```python
from build123d import *

# Parameters (mm, degrees)
SKETCH1_W           = 50
SKETCH1_H           = 37
BOSS_EXTRUDE1_DEPTH = 4
CHAMFER1_SIZE       = 10
SKETCH2_W           = 6
SKETCH2_H           = 37
BOSS_EXTRUDE2_DEPTH = 6
SKETCH3_W           = 37
SKETCH3_H           = 4
BOSS_EXTRUDE3_DEPTH = 40
FILLET1_R           = 10
SKETCH4_R           = 2
CUT_EXTRUDE1_DEPTH  = 40
SKETCH5_R           = 3.25
CUT_EXTRUDE2_DEPTH  = 40
SKETCH6_R           = 7.5
CUT_EXTRUDE3_DEPTH  = 5
SKETCH7_R           = 1.5
CUT_EXTRUDE4_DEPTH  = 9
FILLET2_R           = 2


with BuildPart() as part:
    # Sketch1 → Boss-Extrude1 (new body)
    with BuildSketch(Plane(origin=(0, 0, 0), x_dir=(1, 0, 0), z_dir=(0, 1, 0))):
        Rectangle(SKETCH1_W, SKETCH1_H)
    extrude(amount=BOSS_EXTRUDE1_DEPTH)

    # Chamfer1
    chamfer1_edges = [part.edges().sort_by_distance(p)[0] for p in [
        (-25, 2, 18.5),
        (-25, 2, -18.5),
    ]]
    chamfer(chamfer1_edges, length=CHAMFER1_SIZE)

    # Sketch2 → Boss-Extrude2 (add)
    with BuildSketch(Plane(origin=(0, 4, 0), x_dir=(1, 0, 0), z_dir=(0, 1, 0))):
        with Locations((22, 0)):
            Rectangle(SKETCH2_W, SKETCH2_H)
    extrude(amount=BOSS_EXTRUDE2_DEPTH)

    # Sketch3 → Boss-Extrude3 (add)
    with BuildSketch(Plane.ZY.offset(-19)):
        with Locations((0, 8)):
            Rectangle(SKETCH3_W, SKETCH3_H)
    extrude(amount=BOSS_EXTRUDE3_DEPTH)

    # Fillet1
    fillet1_edges = [part.edges().sort_by_distance(p)[0] for p in [
        (-21, 8, -18.5),
        (-21, 8, 18.5),
    ]]
    fillet(fillet1_edges, radius=FILLET1_R)

    # Sketch4 → Cut-Extrude1 (cut)
    with BuildSketch(Plane(origin=(0, 10, 0), x_dir=(1, 0, 0), z_dir=(0, 1, 0))):
        with Locations(Location((-9, -8.5, 0), (0, 0, 270))):
            Circle(SKETCH4_R)
        with Locations(Location((-9, 8.5, 0), (0, 0, 270))):
            Circle(SKETCH4_R)
    extrude(amount=-CUT_EXTRUDE1_DEPTH, mode=Mode.SUBTRACT)

    # Sketch5 → Cut-Extrude2 (cut)
    with BuildSketch(Plane(origin=(0, 10, 0), x_dir=(1, 0, 0), z_dir=(0, 1, 0))):
        with Locations(Location((8.102581703, 0, 0), (0, 0, 270))):
            Circle(SKETCH5_R)
    extrude(amount=-CUT_EXTRUDE2_DEPTH, mode=Mode.SUBTRACT)

    # Sketch6 → Cut-Extrude3 (cut)
    with BuildSketch(Plane.XZ):
        with Locations(Location((8.102581703, 0, 0), (0, 0, 270))):
            Circle(SKETCH6_R)
    extrude(amount=-CUT_EXTRUDE3_DEPTH, mode=Mode.SUBTRACT)

    # Sketch7 → Cut-Extrude4 (cut)
    with BuildSketch(Plane(origin=(0, 10, 0), x_dir=(1, 0, 0), z_dir=(0, 1, 0))):
        with Locations(Location((22.2, 13.5, 0), (0, 0, 270))):
            Circle(SKETCH7_R)
        with Locations(Location((22.2, 4.5, 0), (0, 0, 270))):
            Circle(SKETCH7_R)
        with Locations(Location((22.2, -4.5, 0), (0, 0, 270))):
            Circle(SKETCH7_R)
        with Locations(Location((22.2, -13.5, 0), (0, 0, 270))):
            Circle(SKETCH7_R)
    extrude(amount=-CUT_EXTRUDE4_DEPTH, mode=Mode.SUBTRACT)

    # Fillet2
    fillet2_edges = [part.edges().sort_by_distance(p)[0] for p in [
        (25, 5, 18.5),
        (25, 5, -18.5),
    ]]
    fillet(fillet2_edges, radius=FILLET2_R)


solid = part.part
```
Check sheet for the modelled part. Datum: model origin and axes. Units: mm. A direction names the side the tool comes from. Coordinates: 2 decimals unless noted, no trailing zeros. Order: outer loops, then holes, each group sorted by start corner. A loop starts at its lowest first (then second) coordinate and runs counter-clockwise, first axis right, second up. Notation, with made-up numbers: (-40, 22.5) -> (4, 22.5) arc R21 ccw to (4, 31.5) -> close; hole circle Ø1 at (10.25, 69). An arc over 180 degrees is marked (long way). Write item = value, one per line. Start each with the question number.
1) Cross-section at C-C (y = 2.25). Enter the section's corners in (x, z).
2) Mould release check, pull along Z, two halves, no side actions. Record for faces 1 (the flat face through (0, 0, 0)), 2 (the cylindrical face through (23.465, 5.563, 5.306)), 3 (the cylindrical face through (24.4, 4.93, -17.93)), 4 (the flat face through (4.3, 3.8, 18.5)): +Z half, -Z half, draft (parallel to the pull), parting line (faces both ways), or undercut.
3) Go/stop test with flat-tipped pins: P1, Ø6, axis at y = 8.5, z = 8.5, coming from the -X side; P2, Ø1, axis at x = 5.5, z = 5, coming from the -Y side; P3, Ø1, axis at y = 5, z = 3, coming from the -X side; P4, Ø6.5, axis at x = -9, z = 8.5, coming from the -Y side. Record where each tip stops, or that it passes through.
4) Cross-section at B-B (z = 4.5). Enter the section's corners in (x, y).
5) Cross-section at D-D (z = -1.5). Enter the section's corners in (x, y), then the cut area to 3 significant figures.
6) Cross-section at A-A (x = -9). Enter the section's corners in (y, z), then the cut area to 3 significant figures.
7) Access from +Z, -Z, +X, -X, +Y, -Y to the whole of each face (thin tool, end or side, straight path). Record for faces 5 (the cylindrical face through (-17.99, 8.03, -15.65)), 6 (the flat face through (22, 1, 13)), 7 (the cylindrical face through (15.54, 1.97, 0.98)), 8 (the flat face through (-1, 6, 0)).
8) Material ranges on L1, parallel to X at y = 1.7, z = 0; L2, parallel to Y at x = -1, z = 3; L3, parallel to X at y = 2.1, z = 8.5, recorded low to high.
Ans:
q1.outline = (-25, -8.5) -> (-15, -18.5) -> (23, -18.5) arc R2 ccw to (25, -16.5) -> (25, 16.5) arc R2 ccw to (23, 18.5) -> (-15, 18.5) -> (-25, 8.5) -> close; hole circle Ø4 at (-9, -8.5); hole circle Ø4 at (-9, 8.5); hole circle Ø15 at (8.1, 0); hole circle Ø3 at (22.2, -13.5); hole circle Ø3 at (22.2, -4.5); hole circle Ø3 at (22.2, 4.5); hole circle Ø3 at (22.2, 13.5)
q2.face_1 = draft
q2.face_2 = undercut
q2.face_3 = -Z half
q2.face_4 = +Z half
q3.P1 = -21
q3.P2 = 6
q3.P3 = 19
q3.P4 = 0
q4.outline = (-25, 0) -> (2.1, 0) -> (2.1, 4) -> (-25, 4) -> close; (-21, 6) -> (19, 6) -> (19, 4) -> (14.1, 4) -> (14.1, 0) -> (25, 0) -> (25, 10) -> (23.7, 10) -> (23.7, 1) -> (20.7, 1) -> (20.7, 10) -> (-21, 10) -> close
q5.outline = (-25, 0) -> (0.75, 0) -> (0.75, 4) -> (-25, 4) -> close; (-21, 6) -> (5.22, 6) -> (5.22, 10) -> (-21, 10) -> close; (10.99, 6) -> (19, 6) -> (19, 4) -> (15.45, 4) -> (15.45, 0) -> (25, 0) -> (25, 10) -> (10.99, 10) -> close
q5.area = 314 mm²
q6.outline = (0, -18.5) -> (4, -18.5) -> (4, -10.5) -> (0, -10.5) -> close; (0, -6.5) -> (4, -6.5) -> (4, 6.5) -> (0, 6.5) -> close; (0, 10.5) -> (4, 10.5) -> (4, 18.5) -> (0, 18.5) -> close; (6, -18.5) -> (10, -18.5) -> (10, -10.5) -> (6, -10.5) -> close; (6, -6.5) -> (10, -6.5) -> (10, 6.5) -> (6, 6.5) -> close; (6, 10.5) -> (10, 10.5) -> (10, 18.5) -> (6, 18.5) -> close
q6.area = 232 mm²
q7.face_5 = -Z, -X, +Y
q7.face_6 = +Y
q7.face_7 = -Y
q7.face_8 = +Z, -Z, -X
q8.L1 = -25 to 0.6, 15.6 to 25
q8.L2 = 0 to 4, 6 to 10
q8.L3 = -25 to -11, -7 to 25
